Autodesk Inventor part; units mm, degrees
ref_plane "YZ Plane" through (0, 0, 0) normal (1, 0, 0) x (0, 1, 0)
ref_plane "XZ Plane" through (0, 0, 0) normal (0, 1, 0) x (-1, 0, 0)
ref_plane "XY Plane" through (0, 0, 0) normal (0, 0, 1) x (1, 0, 0)
sketch "Sketch1" plane through (0, 0, 0) normal (0, 1, 0) x (-1, 0, 0)
  circle A0 centre (0, 0) radius 10.16
  dimension "d0" = 20.32
extrude "Extrusion1" add sketch "Sketch1" along normal blind 304.8
sketch "Sketch2" plane through (0, 304.8, 0) normal (0, 1, 0) x (1, 0, 0)
  line L0 (12.7, -12.7) -> (-12.7, -12.7)
  line L1 (-12.7, -12.7) -> (-12.7, 12.7)
  line L2 (-12.7, 12.7) -> (12.7, 12.7)
  line L3 (12.7, 12.7) -> (12.7, -12.7)
  point P0 (0, 0)
  point P1 (0, 0)
  dimension "d3" = 25.4
  dimension "d4" = 25.4
extrude "Extrusion2" add sketch "Sketch2" along normal blind 25.4
sketch "Sketch3" plane through (12.7, 304.8, -12.7) normal (0, 0, -1) x (-1, 0, 0)
  line L0 (25.4, 0) -> (25.4, 25.4)
  line L1 (0, 0) -> (0, 25.4)
  circle A0 centre (12.7, 12.7) radius 6.35
  point P0 (12.7, -304.8)
  dimension "d7" = 12.7
extrude "Extrusion3" cut sketch "Sketch3" against normal blind 33.3375
fillet "Fillet1" radius 4.7625 2 edges at (0, 330.2, -12.7) (0, 330.2, 12.7)
properties part number "CylinderRod"
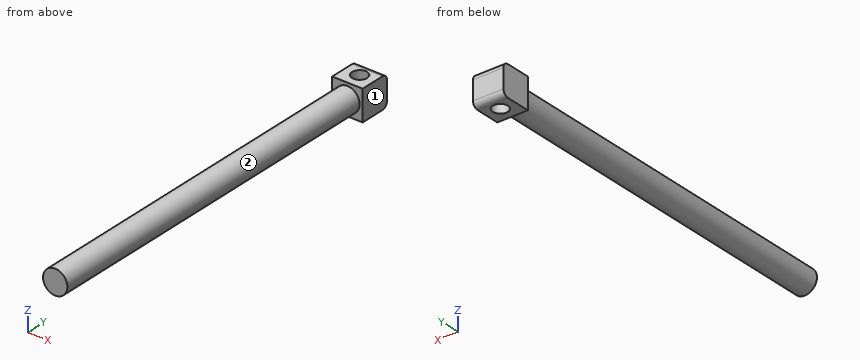
Geometry: final body of the model. Coordinates: model frame, mm. Face numbers are marked on the shaded views. A direction names the side the tool comes from. Round coordinates to 2 decimals unless told otherwise and drop trailing zeros. Loops run counter-clockwise (first coordinate to the right, second up) from the corner with the lowest first, then second, coordinate; pieces in that order, holes last. Notation, with made-up numbers: (21.25, -12) -> (46.25, -12) arc R20 ccw to (46.25, 2) -> close; hole circle Ø8 at (84.5, 82.5). An arc over 180 degrees is marked (long way). Write each question's results on one line, items separated by ' | '.
Item 1: Set-up query: the marked faces 1 and 2. Return all of +Z, -Z, +X, -X, +Y, -Y with unobstructed straight access to the full face (end or side cutting, diameter ignored); none if empty.
Answers below:
face 1: +Z, -Z, +X, +Y, -Y | face 2: -Y
Item 2: Cut plane C-C on y = 317.5. Return the cut outline in (x, z).
Answers below:
outline: (-12.7, -12.7) -> (-6.35, -12.7) -> (-6.35, 12.7) -> (-12.7, 12.7) -> close; (6.35, -12.7) -> (12.7, -12.7) -> (12.7, 12.7) -> (6.35, 12.7) -> close
Item 3: Cut plane D-D on y = 34. Return the cut outline in (x, z).
Answers below:
outline: circle Ø20.32 at (0, 0)
Item 4: Line query: probe 1 along X at (y, z) = (317.5, 6.25); probe 2 along Y at (x, z) = (0, -3.25); probe 3 along Y at (x, z) = (9.5, -8). Output: solid intervals per line, ascending. Write a range as [from, to].
Answers below:
probe 1: x = [-12.7, -6.35], [6.35, 12.7] | probe 2: y = [0, 311.15], [323.85, 330.2] | probe 3: y = [304.8, 330.2]
Item 5: Pin query (flat end, axial travel): pin 1 Ø12 at (x, y) = (8.5, 288.5) entering from -Z; pin 2 Ø8 at (y, z) = (217.5, 2) entering from -X; pin 3 Ø1.5 at (y, z) = (202, -1.5) entering from -X. Return the tip coordinate at first contact, or that it passes through.
Answers below:
pin 1: stops at z = -9.85 | pin 2: stops at x = -10.16 | pin 3: stops at x = -10.13
Item 6: Cut plane B-B on z = 0. Return the cut outline in (x, y), and give its area (3 significant figures).
Answers below:
outline: (-12.7, 304.8) -> (-10.16, 304.8) -> (-10.16, 0) -> (10.16, 0) -> (10.16, 304.8) -> (12.7, 304.8) -> (12.7, 330.2) -> (-12.7, 330.2) -> close; hole circle Ø12.7 at (0, 317.5) | area: 6,710 mm²
